Autodesk Inventor part; units mm, degrees
ref_plane "YZ Plane" through (0, 0, 0) normal (1, 0, 0) x (0, 1, 0)
ref_plane "XZ Plane" through (0, 0, 0) normal (0, 1, 0) x (-1, 0, 0)
ref_plane "XY Plane" through (0, 0, 0) normal (0, 0, 1) x (1, 0, 0)
sketch "Sketch1" plane through (0, 0, 0) normal (0, 1, 0) x (-1, 0, 0)
  line L0 (85, 30) -> (-85, 30)
  line L1 (-85, 30) -> (-85, -30)
  line L2 (-85, -30) -> (85, -30)
  line L3 (85, -30) -> (85, 30)
  line L4 (85, 30) -> (-85, -30) construction
  line L5 (-85, 30) -> (85, -30) construction
  line L6 (0, -42) -> (0, 42)
  point P0 (0, 0)
  point P1 (-100, -30)
  point P2 (-85, -27)
  dimension "d0" = 170
  dimension "d1" = 60
  dimension "d32" = 15
extrude "Extrusion1" add sketch "Sketch1" along normal blind 3
sketch "Sketch2" plane through (0, 3, 0) normal (0, 1, 0) x (1, 0, 0)
  line L0 (-85, 30) -> (-85, -30)
  line L1 (-85, -30) -> (85, -30)
  line L2 (85, -30) -> (85, 30)
  line L3 (80, -25) -> (-80, -25)
  line L4 (-80, -25) -> (-80, 25)
  line L5 (-80, 25) -> (80, 25)
  line L6 (80, 25) -> (80, -25)
  line L7 (80, -25) -> (-80, 25) construction
  line L8 (-80, -25) -> (80, 25) construction
  line L9 (85, 30) -> (-85, 30)
  point P0 (0, 0)
  dimension "d36" = 160
  dimension "d37" = 50
extrude "Extrusion2" add sketch "Sketch2" along normal blind 28
sketch "Sketch9" plane through (-80, 20, 19) normal (1, 0, 0) x (0, 0, -1)
  circle A0 centre (2, -3) radius 3.5
  line L0 (49, -20) -> (-11, -20)
  line L1 (-11, -20) -> (-11, 11)
  point P0 (19, -20)
  point P1 (44, -20)
  dimension "d27" = 7
  dimension "d28" = 17
  dimension "d41" = 13
extrude "Extrusion7" cut sketch "Sketch9" against normal up to surface (5 mm away)
mirror "Mirror2" about plane through (0, 0, 0) normal (1, 0, 0) of "Extrusion7"
sketch "Sketch14" plane through (0, 3, 0) normal (0, 1, 0) x (1, 0, 0)
  point P0 (0, 0)
sketch "Sketch15" plane through (85, 0, 30) normal (1, 0, 0) x (0, 0, -1)
  line L0 (60, 31) -> (0, 31)
  line L1 (60, 31) -> (120, 0)
  line L2 (120, 0) -> (60, 0)
  circle A0 centre (13, 17) radius 3.5
  line L3 (0, 0) -> (60, 0)
  line L4 (60, 0) -> (60, 31)
  line L5 (0, 31) -> (60, 31)
  line L6 (0, 0) -> (0, 31)
  point P0 (30, 0)
  dimension "d67" = 60
extrude "Extrusion12" add sketch "Sketch15" against normal blind 5 contours L1 L2 L4
mirror "Mirror5" about plane through (0, 0, 0) normal (1, 0, 0) of "Extrusion12"
equation "\"d0\" = Width"
equation "\"d1\" = Length"
equation "\"d2\" = BaseWallThickness"
equation "\"d36\" = Width - 2 * SideWallThickness"
equation "\"d37\" = Length - 2 * SideWallThickness"
equation "\"d5\" = Height - 2 * BaseWallThickness"
equation "\"d28\" = DriveMotorHeight"
equation "\"d67\" = WedgeLength"
equation "\"d68\" = SideWallThickness"
equation "\"SideWallThickness\" = 5"
equation "\"BaseWallThickness\" = 3"
equation "\"Width\" = 170"
equation "\"Length\" = 60"
equation "\"Height\" = 34"
equation "\"DriveMotorHeight\" = 17"
equation "\"DriveMotorMountThickness\" = 2"
equation "\"WedgeLength\" = 60"
properties part number "BodyWedgeV1-NoMotor" material "Thermoplastic Resin"
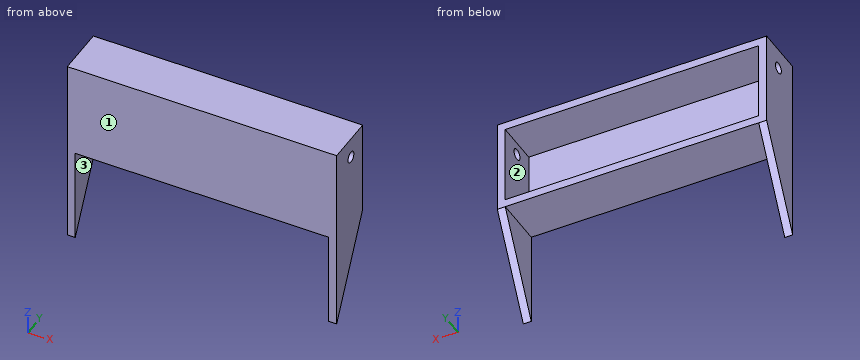
Model file for the job. Use its own axes, mm. Face numbers are marked on the shaded views. A direction names the side the tool comes from. Give positions to 0.01 mm unless a question says otherwise; leave off trailing zeros. Order: outer loops, then holes, each group sorted by start corner. A loop starts at its lowest first (then second) coordinate and runs counter-clockwise, first axis right, second up. Notation, with made-up numbers: (22.25, 1) - (35.25, 1) arc R25 cw to (35.25, 39) - close; hole circle Ø9 at (70, -13.75). An arc over 180 degrees is marked (long way). One line per item, written item: value.
Item 1: Slice it at D-D (x = 51.5). List the corners of the cut face in (y, z).
Response values:
outline: (0, -30) - (31, -30) - (31, -25) - (3, -25) - (3, 25) - (31, 25) - (31, 30) - (0, 30) - close
Item 2: Slice it at C-C (y = 6.5). List the corners of the cut face in (x, z).
Response values:
outline: (-85, -77.42) - (-80, -77.42) - (-80, -30) - (80, -30) - (80, -77.42) - (85, -77.42) - (85, 30) - (-85, 30) - close; hole (-80, -25) - (80, -25) - (80, 25) - (-80, 25) - close
Item 3: Slice it at A-A (z = 17). List the corners of the cut face in (x, y), then the cut area to 3 significant figures.
Response values:
outline: (-85, 0) - (85, 0) - (85, 13.5) - (80, 13.5) - (80, 3) - (-80, 3) - (-80, 13.5) - (-85, 13.5) - close; (-85, 20.5) - (-80, 20.5) - (-80, 31) - (-85, 31) - close; (80, 20.5) - (85, 20.5) - (85, 31) - (80, 31) - close
area: 720 mm2
Item 4: Pin check, flat tips, straight feed: pin 1 Ø10 at (x, y) = (-52, 6) entering from -Z; pin 2 Ø4 at (x, z) = (62.5, -10.5) entering from +Y; pin 3 Ø6.5 at (y, z) = (17, 17) entering from -X. Stop position of each tip, or through.
Response values:
pin 1: z = -30
pin 2: y = 3
pin 3: through
Item 5: Tool access for the marked faces 1, 2 and 3: list every direction of +Z, -Z, +X, -X, +Y, -Y with a clear straight run to the whole face (end or side of a thin tool).
Response values:
face 1: +Z, -Z, +X, -X, -Y
face 2: +Y
face 3: -Z, +Y, -Y
Item 6: Slice it at B-B (y = 17). List the corners of the cut face in (x, z).
Response values:
outline: (-85, -57.1) - (-80, -57.1) - (-80, -30) - (80, -30) - (80, -57.1) - (85, -57.1) - (85, 13.5) - (80, 13.5) - (80, -25) - (-80, -25) - (-80, 13.5) - (-85, 13.5) - close; (-85, 20.5) - (-80, 20.5) - (-80, 25) - (80, 25) - (80, 20.5) - (85, 20.5) - (85, 30) - (-85, 30) - close
Item 7: Wall check: line 1 (X direction, y = 12.5, z = 7.5); line 2 (Z direction, x = -30.5, y = 17.5); line 3 (Y direction, x = -81.35, z = 17). Give the ranges that are in metal, low to high.
Response values:
line 1: -85 to -80, 80 to 85
line 2: -30 to -25, 25 to 30
line 3: 0 to 13.5, 20.5 to 31
